Geometry: see drawing. Coordinates: mm, zero at the bounding-box minimum. Give positions to 0.01 mm unless a question says otherwise; leave off trailing zeros. Loops run counter-clockwise (first coordinate to the right, second up) from the corner with the lowest first, then second, coordinate; pieces in that order, holes last. Notation, with made-up numbers: (22, -2.5) -> (79, -2.5) arc R30 ccw to (79, 21.5) -> close; hole circle Ø5 at (87.5, -35). An arc over 180 degrees is marked (long way). Answer in a Markdown table with one row per item. Add a question column.
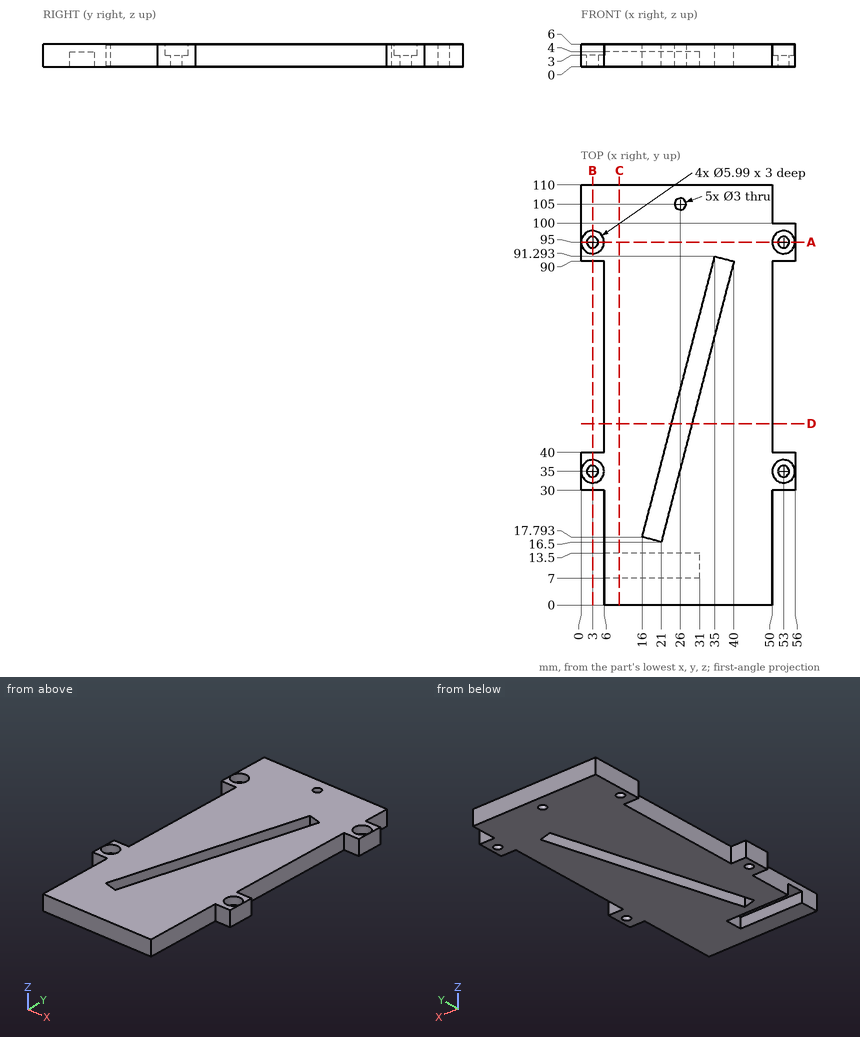
1) Section A-A on y = 95. State how many separate pieces and enclosed holes the cut face has, and give its area (3 significant figures).
2) Pin query (flat end, axial travel): pin 1 (6 mm diameter, centred on x = 50, y = 86, fed in from -Z); pin 2 (1.2 mm diameter, centred on y = 11, z = 1, fed in from -X); pin 3 (1.8 mm diameter, centred on x = 54, z = 3, fed in from +Y); pin 4 (3 mm diameter, centred on y = 48.5, z = 4, fed in from -X). Return the tip coordinate at first contact, or that it passes through.
3) Section D-D on y = 47.5. Output: boundary loops of the cut face in (x, z), and give its area (3 significant figures).
4) Material intervals for line 1 along X through (y, z) = (95, 2.3); line 2 along Y through (x, z) = (53, 3.8) (1 decimal); line 3 along Y through (x, z) = (3, 2.2), sorted ascending.
5) Section B-B on x = 3. Output: boundary loops of the cut face in (y, z) (1 decimal).
6) Section C-C on x = 10. Output: boundary loops of the cut face in (y, z), and give its area (3 significant figures).
Working result:
| question | item | result |
|---|---|---|
| 1 | separate pieces | 3 |
| 1 | enclosed holes | 0 |
| 1 | area | 282 mm2 |
| 2 | pin 1 | stops at z = 0 |
| 2 | pin 2 | stops at x = 31 |
| 2 | pin 3 | stops at y = 100 |
| 2 | pin 4 | stops at x = 6 |
| 3 | outline | (6, 0) -> (23.68, 0) -> (23.68, 6) -> (6, 6) -> close; (29.01, 0) -> (50, 0) -> (50, 6) -> (29.01, 6) -> close |
| 3 | area | 232 mm2 |
| 4 | line 1 | x = 0 to 1.5, 4.5 to 51.5, 54.5 to 56 |
| 4 | line 2 | y = 30 to 32, 38 to 40, 90 to 92, 98 to 100 |
| 4 | line 3 | y = 30 to 33.5, 36.5 to 40, 90 to 93.5, 96.5 to 110 |
| 5 | outline | (30, 0) -> (33.5, 0) -> (33.5, 3) -> (32, 3) -> (32, 6) -> (30, 6) -> close; (36.5, 0) -> (40, 0) -> (40, 6) -> (38, 6) -> (38, 3) -> (36.5, 3) -> close; (90, 0) -> (93.5, 0) -> (93.5, 3) -> (92, 3) -> (92, 6) -> (90, 6) -> close; (96.5, 0) -> (110, 0) -> (110, 6) -> (98, 6) -> (98, 3) -> (96.5, 3) -> close |
| 6 | outline | (0, 0) -> (7, 0) -> (7, 4) -> (13.5, 4) -> (13.5, 0) -> (110, 0) -> (110, 6) -> (0, 6) -> close |
| 6 | area | 634 mm2 |
